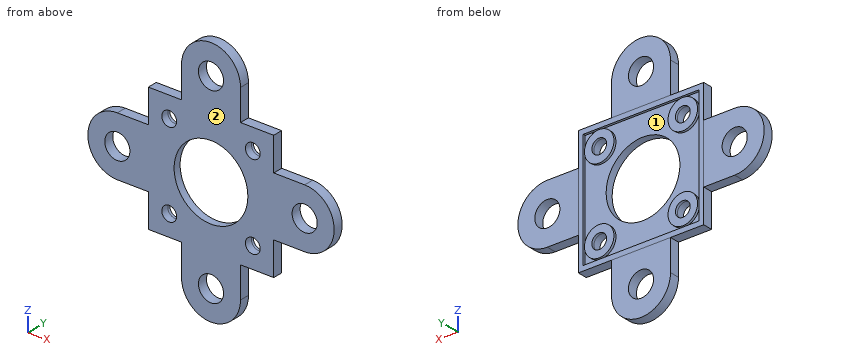
```python
from build123d import *

# Parameters (mm, degrees)
SKETCH1_W           = 23
SKETCH1_H           = 23
SKETCH1_R           = 1.5
BOSS_EXTRUDE1_DEPTH = 1
SKETCH2_W           = 6
SKETCH2_H           = 5
BOSS_EXTRUDE2_DEPTH = 1
FILLET1_R           = 3
BOSS_EXTRUDE3_START = -3
SKETCH3_W           = 25.5
SKETCH3_H           = 25.5
SKETCH3_R           = 1.5
SKETCH3_R_2         = 7.5
BOSS_EXTRUDE3_DEPTH = 1.5
SKETCH4_R           = 3
SKETCH4_R_2         = 1.5
BOSS_EXTRUDE4_DEPTH = 2
SKETCH5_W           = 25.5
SKETCH5_H           = 25.5
SKETCH5_W_2         = 23.5
SKETCH5_H_2         = 23.5
BOSS_EXTRUDE5_DEPTH = 2
SKETCH6_R           = 2.5527
BOSS_EXTRUDE6_DEPTH = 2
CIRPATTERN1_COUNT   = 4


with BuildPart() as part:
    # Sketch1 → Boss-Extrude1 (new body)
    with BuildSketch(Plane(origin=(0, 0, 0), x_dir=(1, 0, 0), z_dir=(0, 1, 0))):
        Rectangle(SKETCH1_W, SKETCH1_H)
        with Locations((-8.5, 8.5)):
            Circle(SKETCH1_R, mode=Mode.SUBTRACT)
        with Locations((8.5, 8.5)):
            Circle(SKETCH1_R, mode=Mode.SUBTRACT)
        with Locations((8.5, -8.5)):
            Circle(SKETCH1_R, mode=Mode.SUBTRACT)
        with Locations((-8.5, -8.5)):
            Circle(SKETCH1_R, mode=Mode.SUBTRACT)
    extrude(amount=BOSS_EXTRUDE1_DEPTH)

    # Sketch2 → Boss-Extrude2 (add)
    with BuildSketch(Plane(origin=(0, 1, 0), x_dir=(1, 0, 0), z_dir=(0, 1, 0))):
        Rectangle(SKETCH2_W, SKETCH2_H)
    extrude(amount=BOSS_EXTRUDE2_DEPTH)

    # Fillet1
    fillet1_edges = [part.edges().sort_by_distance(p)[0] for p in [
        (11.5, 0.5, 11.5),
        (-11.5, 0.5, 11.5),
        (-11.5, 0.5, -11.5),
        (11.5, 0.5, -11.5),
    ]]
    fillet(fillet1_edges, radius=FILLET1_R)


with BuildPart() as body_2:
    # Sketch3 → Boss-Extrude3 (new body)
    with BuildSketch(Plane(origin=(0, 1, 0), x_dir=(1, 0, 0), z_dir=(0, 1, 0)).offset(BOSS_EXTRUDE3_START)):
        Rectangle(SKETCH3_W, SKETCH3_H)
        with Locations((-8.5, 8.5)):
            Circle(SKETCH3_R, mode=Mode.SUBTRACT)
        with Locations((8.5, 8.5)):
            Circle(SKETCH3_R, mode=Mode.SUBTRACT)
        with Locations((8.5, -8.5)):
            Circle(SKETCH3_R, mode=Mode.SUBTRACT)
        with Locations((-8.5, -8.5)):
            Circle(SKETCH3_R, mode=Mode.SUBTRACT)
        Circle(SKETCH3_R_2, mode=Mode.SUBTRACT)
    extrude(amount=BOSS_EXTRUDE3_DEPTH)

    # Sketch4 → Boss-Extrude4 (add)
    with BuildSketch(Plane.XZ.offset(2)):
        with Locations((-8.5, 8.5)):
            Circle(SKETCH4_R)
        with Locations((-8.5, 8.5)):
            Circle(SKETCH4_R_2, mode=Mode.SUBTRACT)
        with Locations((8.5, 8.5)):
            Circle(SKETCH4_R)
        with Locations((8.5, 8.5)):
            Circle(SKETCH4_R_2, mode=Mode.SUBTRACT)
        with Locations((8.5, -8.5)):
            Circle(SKETCH4_R)
        with Locations((8.5, -8.5)):
            Circle(SKETCH4_R_2, mode=Mode.SUBTRACT)
        with Locations((-8.5, -8.5)):
            Circle(SKETCH4_R)
        with Locations((-8.5, -8.5)):
            Circle(SKETCH4_R_2, mode=Mode.SUBTRACT)
    extrude(amount=-BOSS_EXTRUDE4_DEPTH)

    # Sketch5 → Boss-Extrude5 (add)
    with BuildSketch(Plane.XZ.offset(2)):
        Rectangle(SKETCH5_W, SKETCH5_H)
        Rectangle(SKETCH5_W_2, SKETCH5_H_2, mode=Mode.SUBTRACT)
    extrude(amount=-BOSS_EXTRUDE5_DEPTH)

    # Sketch6 → Boss-Extrude6 (add)
    with BuildSketch(Plane(origin=(0, 0, 0), x_dir=(-1, 0, 0), z_dir=(0, 1, 0))):
        with BuildLine():
            Line((-6, -19.05), (-6, -12.75))
            Line((-6, -12.75), (6, -12.75))
            Line((6, -12.75), (6, -19.05))
            ThreePointArc((6, -19.05), (0, -25.05), (-6, -19.05))
        make_face()
        with Locations((0, -19.05)):
            Circle(SKETCH6_R, mode=Mode.SUBTRACT)
    boss_extrude6 = extrude(amount=-BOSS_EXTRUDE6_DEPTH)

    # CirPattern1: Boss-Extrude6 ×4 about axis
    cirpattern1_axis = Axis((0, 0, 0), (0, 1, 0))
    for i in range(1, CIRPATTERN1_COUNT):
        add(boss_extrude6.rotate(cirpattern1_axis, i * 360 / CIRPATTERN1_COUNT))


solid = body_2.part
```
Verification items for the finished model (mm, model axes). Face numbers are marked on the shaded views. Give positions to 0.01 mm unless a question says otherwise; leave off trailing zeros. Order: outer loops, then holes, each group sorted by start corner. A loop starts at its lowest first (then second) coordinate and runs counter-clockwise, first axis right, second up. Notation, with made-up numbers: M 88.25,41.25 L 138.25,41.25 A17 ccw 138.25,56.25 Z; hole C 78,-28 d3. An arc over 180 degrees is marked long. Answer in a Markdown table with one row per item. Add a question column.
Item 1: Section check C-C, the plane y = -1.65. State how many separate pieces and enclosed holes the cut face has, and give its area (3 significant figures).
Item 2: Section check A-A, the plane x = 0. Enter the section's corners in (y, z), and give its area (3 significant figures).
Item 3: Section check D-D, the plane x = 8.5. Enter the section's corners in (y, z).
Item 4: Section check B-B, the plane z = 0. Enter the section's corners in (x, y).
Item 5: Scan lines: probe 1 along X at (y, z) = (-1.25, -8.5); probe 2 along Z at (x, y) = (-8.5, -0.2); probe 3 along Z at (x, y) = (0, -1.55). Record each from-to range of solid material in increasing order. Write a range as from..to.
Item 6: Gauge pin test, flat ends, axial feed: pin 1 (0.6 mm diameter, centred on y = -0.5, z = -4.5, fed in from +X); pin 2 (1 mm diameter, centred on y = -1.5, z = 19, fed in from +X); pin 3 (1 mm diameter, centred on y = -1, z = 5, fed in from -X). Record the tip position at first contact, or that the pin passes through.
Item 7: Mould release check, pull along X, two halves, no side actions. Record for the marked faces 1 and 2: released by +X, released by -X, zero draft, split by the parting line, or undercut.
Filled sheet:
| question | item | result |
|---|---|---|
| 1 | separate pieces | 1 |
| 1 | enclosed holes | 9 |
| 1 | area | 892 mm^2 |
| 2 | outline | M -2,-25.05 L 0,-25.05 L 0,-21.6 L -2,-21.6 Z; M -2,-16.5 L 0,-16.5 L 0,-11.75 L -0.5,-11.75 L -0.5,-7.5 L -2,-7.5 Z; M -2,7.5 L -0.5,7.5 L -0.5,11.75 L 0,11.75 L 0,16.5 L -2,16.5 Z; M -2,21.6 L 0,21.6 L 0,25.05 L -2,25.05 Z |
| 2 | area | 45.5 mm^2 |
| 3 | outline | M -2,-12.75 L 0,-12.75 L 0,-11.75 L -0.5,-11.75 L -0.5,-11.5 L 0,-11.5 L 0,-10 L -2,-10 Z; M -2,-7 L 0,-7 L 0,-5.5 L -0.5,-5.5 L -0.5,5.5 L 0,5.5 L 0,7 L -2,7 Z; M -2,10 L 0,10 L 0,11.5 L -0.5,11.5 L -0.5,11.75 L 0,11.75 L 0,12.75 L -2,12.75 Z |
| 4 | outline | M -25.05,-2 L -21.6,-2 L -21.6,0 L -25.05,0 Z; M -16.5,-2 L -7.5,-2 L -7.5,-0.5 L -11.75,-0.5 L -11.75,0 L -16.5,0 Z; M 7.5,-2 L 16.5,-2 L 16.5,0 L 11.75,0 L 11.75,-0.5 L 7.5,-0.5 Z; M 21.6,-2 L 25.05,-2 L 25.05,0 L 21.6,0 Z |
| 5 | probe 1 | x = -12.75..-10, -7..7, 10..12.75 |
| 5 | probe 2 | z = -12.75..-11.75, -11.5..-10, -7..-5.5, 5.5..7, 10..11.5, 11.75..12.75 |
| 5 | probe 3 | z = -25.05..-21.6, -16.5..-7.5, 7.5..16.5, 21.6..25.05 |
| 6 | pin 1 | stops at x = 23.33 |
| 6 | pin 2 | stops at x = 6 |
| 6 | pin 3 | stops at x = -23.02 |
| 7 | face 1 | undercut |
| 7 | face 2 | zero draft |
